Here's how the part is built. I have some questions about the finished solid (model axes, mm). Face numbers are marked on the shaded views. A direction names the side the tool comes from. Round coordinates to 2 decimals unless told otherwise and drop trailing zeros. Order: outer loops, then holes, each group sorted by start corner. A loop starts at its lowest first (then second) coordinate and runs counter-clockwise, first axis right, second up. Notation, with made-up numbers: (9, 79) - (45, 79) arc R22 cw to (45, 108) - close; hole circle Ø8 at (84.25, 76.25). An arc over 180 degrees is marked (long way). One line per item, written item: value.
from build123d import *

# Parameters (mm, degrees)
SKETCH1_R           = 12
BOSS_EXTRUDE1_DEPTH = 8
SKETCH2_R           = 2.05
CUT_EXTRUDE1_DEPTH  = 9
CUT_EXTRUDE2_DEPTH  = 9
CIRPATTERN1_COUNT   = 18


with BuildPart() as part:
    # Sketch1 → Boss-Extrude1 (new body)
    with BuildSketch(Plane(origin=(0, 0, 0), x_dir=(1, 0, 0), z_dir=(0, 1, 0))):
        Circle(SKETCH1_R)
    extrude(amount=BOSS_EXTRUDE1_DEPTH)

    # Sketch2 → Cut-Extrude1 (cut, through all)
    with BuildSketch(Plane(origin=(0, 8, 0), x_dir=(1, 0, 0), z_dir=(0, 1, 0))):
        Circle(SKETCH2_R)
    extrude(amount=-CUT_EXTRUDE1_DEPTH, mode=Mode.SUBTRACT)

    # Sketch3 → Cut-Extrude2 (cut, through all)
    with BuildSketch(Plane(origin=(0, 8, 0), x_dir=(1, 0, 0), z_dir=(0, 1, 0))):
        Polygon((0, 8.5), (0.5, 8.5), (1.5, 11.9058809), (1.5, 12.741082781), (-1.5, 12.741082781), (-1.5, 11.9058809), (-0.5, 8.5), align=None)
    cut_extrude2 = extrude(amount=-CUT_EXTRUDE2_DEPTH, mode=Mode.SUBTRACT)

    # CirPattern1: Cut-Extrude2 ×18 about axis
    cirpattern1_axis = Axis((0, 0, 0), (0, 1, 0))
    for i in range(1, CIRPATTERN1_COUNT):
        add(cut_extrude2.rotate(cirpattern1_axis, i * 360 / CIRPATTERN1_COUNT), mode=Mode.SUBTRACT)


solid = part.part
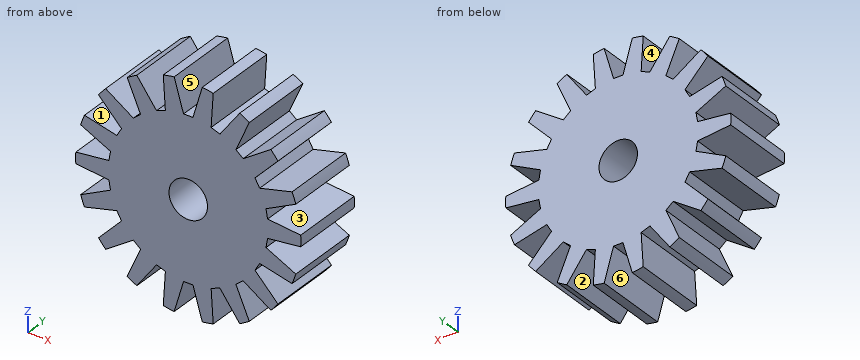
Q1. If we section it at C-C, the plane x = -10: Please give me the cut outline in (y, z).
Results list:
outline: (0, -4.4) - (8, -4.4) - (8, -2.82) - (0, -2.82) - close; (0, -0.81) - (8, -0.81) - (8, 0.81) - (0, 0.81) - close; (0, 2.82) - (8, 2.82) - (8, 4.4) - (0, 4.4) - close
Q2. If we section it at B-B, the plane z = 0: Please give me the cut outline in (x, y), then the cut area to 3 significant figures.
Results list:
outline: (-12, 0) - (-2.05, 0) - (-2.05, 8) - (-12, 8) - close; (2.05, 0) - (12, 0) - (12, 8) - (2.05, 8) - close
area: 159 mm²
Q3. If we section it at D-D, the plane z = 2.75: Please give me the cut outline in (x, y).
Results list:
outline: (-9.86, 0) - (9.86, 0) - (9.86, 8) - (-9.86, 8) - close
Q4. We'd pull the mould along Z, two halves only. Please class the marked faces 4, 5 and 6: released by +Z, released by -Z, zero draft, split by the parting line, or undercut.
Results list:
face 4: undercut
face 5: released by +Z
face 6: released by -Z
Q5. Will these pins go through, and if not, where does the flat tip stop? pin 1 (0.8 mm diameter, centred on x = 0, y = 2.5, fed in from +Z); pin 2 (4 mm diameter, centred on x = 7, y = 2, fed in from -Z); pin 3 (4 mm diameter, centred on y = 2, z = -4.5, fed in from +X).
Results list:
pin 1: z = 8.5
pin 2: z = -10.67
pin 3: x = 11.46
Q6. If we section it at A-A, the plane x = 0: Please give me the cut outline in (y, z).
Results list:
outline: (0, -8.5) - (8, -8.5) - (8, -2.05) - (0, -2.05) - close; (0, 2.05) - (8, 2.05) - (8, 8.5) - (0, 8.5) - close
Q7. If I drill on line 1 along X through (y, z) = (6.5, -8.25); line 2 along X through (y, z) = (4.5, -7.75); line 3 along Z through (x, y) = (-7.25, 7.5), over which ranges is the centre line in solid material (lowest first)?
Results list:
line 1: -5.7 to -3.7, -2.44 to 2.44, 3.7 to 5.7
line 2: -9.16 to -8.19, -5.48 to 5.48, 8.19 to 9.16
line 3: -7.12 to -4.83, -4.44 to 4.44, 4.83 to 7.12
Q8. Which directions (+Z, -Z, +X, -X, +Y, -Y) give clear straight access to the entire face, cutting with the end or side of a thin tool? Please do the marked faces 1, 2 and 3.
Results list:
face 1: +Y, -Y
face 2: -Z, +Y, -Y
face 3: +X, +Y, -Y
